Drawing for the job (mm, zero at the part's lowest x, y, z). A direction names the side the tool comes from. Coordinates: 2 decimals unless noted, no trailing zeros. Write each loop counter-clockwise with the first axis right and the second up, starting at its lowest first coordinate (ties: lowest second). Pieces come first, ordered by that corner, then holes. Notation, with made-up numbers: (38, -33) -> (76, -33) arc R24 cw to (76, 6) -> close; hole circle Ø6 at (53.5, 51). An arc over 180 degrees is marked (long way). Write each question's results on one line, items separated by ' | '. Start each with the question number.
Q1. Saw through at D-D on x = 28. Give the cut face in (y, z) (1 decimal).
Q2. Saw through at B-B on z = 12.25. Give the cut face in (x, y) (1 decimal).
Q3. Tool access for the marked faces 1 and 2: list every direction of +Z, -Z, +X, -X, +Y, -Y with a clear straight run to the whole face (end or side of a thin tool).
Q4. Saw through at C-C on y = 11.75. Give the cut face in (x, z).
Q5. Two-plate mould, pull along X, no slides. Class the marked faces 3, 4 and 5: released by +X, released by -X, zero draft, split by the parting line, or undercut.
Q6. Drill centre lines: line 1 (Y direction, x = 8, z = 14.5); line 2 (Y direction, x = 11, z = 12); line 3 (X direction, y = 14.25, z = 19.5) (1 decimal). Where is each one in solid material? Low to high.
Q7. Saw through at A-A on x = 32.5. Give the cut face in (y, z).
Q8. Drop flat-ended pins along their axis: pin 1 Ø3 at (x, z) = (8.5, 12.5) entering from +Y; pin 2 Ø10 at (y, z) = (15.5, 10.5) entering from +X; pin 3 Ø3 at (x, y) = (21.5, 21) entering from -Z (1 decimal); pin 4 Ø3 at (x, z) = (32, 13.25) entering from +Y. Give the stop position or say it passes through.
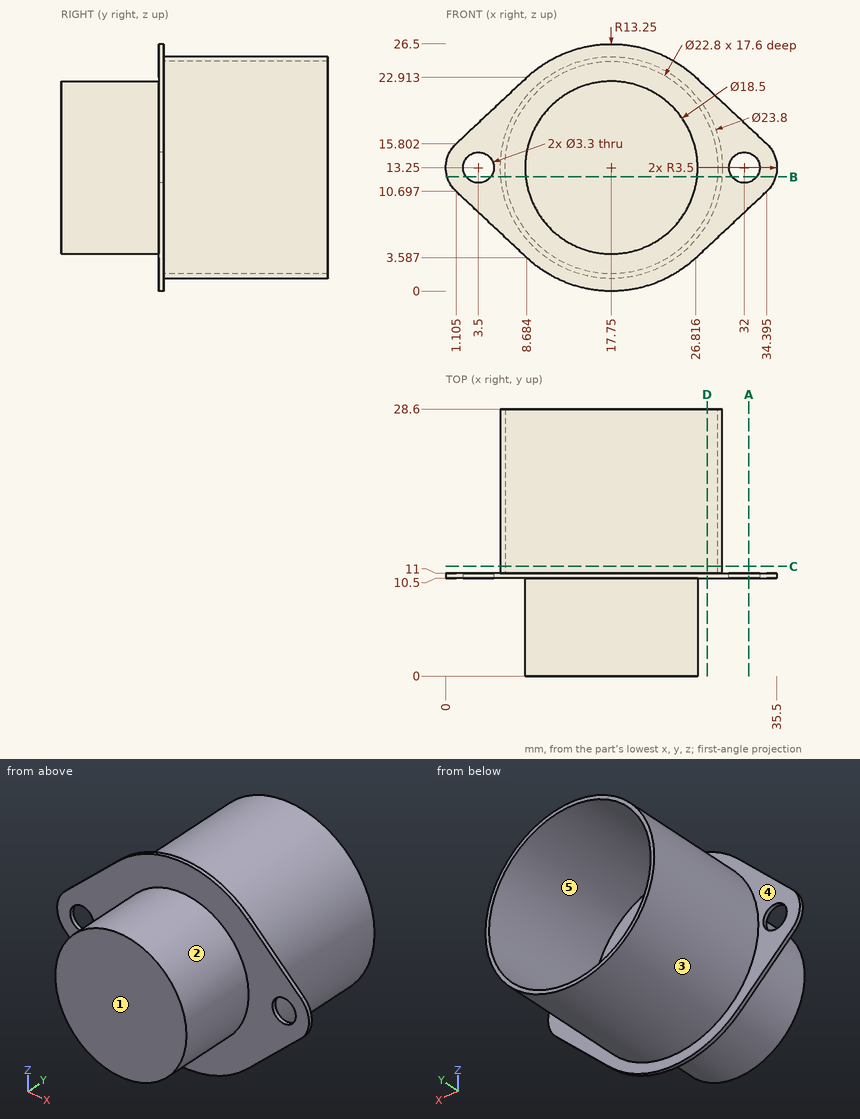
Returned:
1) outline: (10.5, 4.7) -> (11, 4.7) -> (11, 7.2) -> (28.6, 7.2) -> (28.6, 8.3) -> (11, 8.3) -> (11, 18.2) -> (28.6, 18.2) -> (28.6, 19.3) -> (11, 19.3) -> (11, 21.8) -> (10.5, 21.8) -> close
2) outline: (0.1, 10.5) -> (2.2, 10.5) -> (2.2, 11) -> (0.1, 11) -> close; (4.8, 10.5) -> (8.6, 10.5) -> (8.6, 0) -> (26.9, 0) -> (26.9, 10.5) -> (30.7, 10.5) -> (30.7, 11) -> (29.6, 11) -> (29.6, 28.6) -> (29.1, 28.6) -> (29.1, 11) -> (6.4, 11) -> (6.4, 28.6) -> (5.9, 28.6) -> (5.9, 11) -> (4.8, 11) -> close; (33.3, 10.5) -> (35.4, 10.5) -> (35.4, 11) -> (33.3, 11) -> close
3) face 1: +Z, -Z, +X, -X, -Y | face 2: -Y
4) outline: circle Ø23.8 at (17.75, 13.25); hole circle Ø22.8 at (17.75, 13.25)
5) face 3: split by the parting line | face 4: zero draft | face 5: undercut
6) line 1: y = 10.5 to 11 | line 2: y = 0 to 11 | line 3: x = 7.6 to 8.2, 27.3 to 27.9
7) outline: (10.5, 8.92) -> (11, 8.92) -> (11, 11.68) -> (10.5, 11.68) -> close; (10.5, 14.82) -> (11, 14.82) -> (11, 17.58) -> (10.5, 17.58) -> close
8) pin 1: stops at y = 11 | pin 2: stops at x = 35.45 | pin 3: stops at z = 1.6 | pin 4: passes through
